Can you work these out from the model? Positions are in its coordinate system, mm. A direction names the side the tool comes from. Coordinates: 2 decimals unless noted, no trailing zeros. Order: outer loops, then holes, each group sorted by start corner. A loop starts at its lowest first (then second) coordinate and runs counter-clockwise, first axis right, second up. Notation, with made-up numbers: (34, 86.5) -> (64, 86.5) arc R22 cw to (64, 96.5) -> close; hole circle Ø4 at (58.5, -28.75). An arc over 180 degrees is marked (long way). Answer in a Markdown table with one row per item. Add a question column.
1. Imagine slicing it at B-B on z = 11.75. Write out the boundary of the cut face in (x, y).
2. If I drill on line 1 along X through (y, z) = (-0.75, 13.75); line 2 along Y through (x, z) = (0, 1.7); line 3 along Z through (x, y) = (0, -11.5), over which ranges is the centre line in solid material (lowest first)? Write a range as [from, to].
3. Will these pins go through, and if not, where does the flat tip stop? pin 1 (8 mm diameter, centred on x = -5, y = 4, fed in from -Z); pin 2 (0.6 mm diameter, centred on x = 8.5, z = 26, fed in from +Y); pin 3 (12 mm diameter, centred on x = 0, z = 20, fed in from +Y); pin 4 (1.6 mm diameter, centred on x = -9, z = 25.5, fed in from +Y).
4. Imagine slicing it at A-A on x = 0. Write out the boundary of the cut face in (y, z).
5. Imagine slicing it at C-C on y = 11.5. Write out the boundary of the cut face in (x, z).
6. Imagine slicing it at D-D on y = 2.25. Write out the boundary of the cut face in (x, z).
7. On a 3-axis mill with a long thin cutter (end or side, diameter ignored), from which of +Z, -Z, +X, -X, +Y, -Y can I reach the whole of each face in a straight line? I mean faces 5 (the face through (1.61, -11.97, 19.45)), 6 (the face through (0, -10, 13)), 7 (the face through (9, -6, 26)). Say none if no direction works.
8. We'd pull the mould along Y, two halves only. Please class faces 1 (the face through (-0.65, -0.01, 2.03)), 2 (the face through (-9, 12, 8)), 3 (the face through (2, -14, 14)), 4 (the face through (-8.682, 13.715, 7.699)): pulls with the +Y half, pulls with the -Y half, needs draft (parallel to the pull), parting line crosses it, or undercut.
from build123d import *

# Parameters (mm, degrees)
SKETCH_1_W          = 20
SKETCH_1_H          = 28
EXTRUDE_1_DEPTH     = 4
SKETCH_2_W          = 20
SKETCH_2_H          = 4
EXTRUDE_2_DEPTH     = 24
EXTRUDE_3_DEPTH     = 2.6
FILLET_1_R          = 1
SKETCH_4_R          = 3
CUT_EXTRUDE_1_DEPTH = 30.52964612


with BuildPart() as part:
    # 草图1 → 凸台-拉伸1 (new body)
    with BuildSketch(Plane.XY):
        Rectangle(SKETCH_1_W, SKETCH_1_H)
    extrude(amount=EXTRUDE_1_DEPTH)

    # 草图2 → 凸台-拉伸2 (add)
    with BuildSketch(Plane.XY.offset(4)):
        with Locations((0, -12)):
            Rectangle(SKETCH_2_W, SKETCH_2_H)
    extrude(amount=EXTRUDE_2_DEPTH)

    # 草图3 → 凸台-拉伸3 (add)
    with BuildSketch(Plane.ZY.offset(10)):
        Polygon((4, 14), (8, 14), (8, 11), (25, -6), (28, -6), (28, -10), (4, -10), align=None)
    extrude_3 = extrude(amount=-EXTRUDE_3_DEPTH)

    # 镜向1: 凸台-拉伸3 across plane
    add(extrude_3.mirror(Plane(origin=(0, 0, 0), x_dir=(0, 0, 1), z_dir=(1, 0, 0))))

    # 圆角1
    fillet_1_edges = [part.edges().sort_by_distance(p)[0] for p in [
        (-8.7, 14, 8),
        (-8.7, -6, 28),
        (8.7, -6, 28),
        (8.7, 14, 8),
    ]]
    fillet(fillet_1_edges, radius=FILLET_1_R)

    # 草图4 → 切除-拉伸1 (cut, through all)
    with BuildSketch(Plane.XY.offset(4)):
        with Locations((0, 2.920534958)):
            Circle(SKETCH_4_R)
    cut_extrude_1 = extrude(amount=-CUT_EXTRUDE_1_DEPTH, mode=Mode.SUBTRACT)

    # 镜向2: 切除-拉伸1 across plane
    add(cut_extrude_1.mirror(Plane(origin=(0, -7, 7), x_dir=(0, 0.7071067811865476, 0.7071067811865476), z_dir=(0, -0.7071067811865477, 0.7071067811865475))), mode=Mode.SUBTRACT)


solid = part.part
Answers follow:
| question | item | result |
|---|---|---|
| 1 | outline | (-10, -14) -> (10, -14) -> (10, 7.25) -> (7.4, 7.25) -> (7.4, -10) -> (-7.4, -10) -> (-7.4, 7.25) -> (-10, 7.25) -> close |
| 2 | line 1 | x = [-10, -7.4], [7.4, 10] |
| 2 | line 2 | y = [-14, -0.08], [5.92, 14] |
| 2 | line 3 | z = [0, 13.92], [19.92, 28] |
| 3 | pin 1 | stops at z = 0 |
| 3 | pin 2 | stops at y = -6 |
| 3 | pin 3 | stops at y = -10 |
| 3 | pin 4 | stops at y = -5.7 |
| 4 | outline | (-14, 0) -> (-0.08, 0) -> (-0.08, 4) -> (-10, 4) -> (-10, 13.92) -> (-14, 13.92) -> close; (-14, 19.92) -> (-10, 19.92) -> (-10, 28) -> (-14, 28) -> close; (5.92, 0) -> (14, 0) -> (14, 4) -> (5.92, 4) -> close |
| 5 | outline | (-10, 0) -> (10, 0) -> (10, 8) -> (7.4, 8) -> (7.4, 4) -> (-7.4, 4) -> (-7.4, 8) -> (-10, 8) -> close |
| 6 | outline | (-10, 0) -> (-2.92, 0) -> (-2.92, 4) -> (-7.4, 4) -> (-7.4, 16.75) -> (-10, 16.75) -> close; (2.92, 0) -> (10, 0) -> (10, 16.75) -> (7.4, 16.75) -> (7.4, 4) -> (2.92, 4) -> close |
| 7 | face 5 | +Y, -Y |
| 7 | face 6 | +Z, +Y |
| 7 | face 7 | +Z, +X, -X, +Y |
| 8 | face 1 | undercut |
| 8 | face 2 | needs draft |
| 8 | face 3 | pulls with the -Y half |
| 8 | face 4 | pulls with the +Y half |
